Build history of the part. All positions in model axes, mm. Face numbers are marked on the shaded views. Round coordinates to 2 decimals unless told otherwise and drop trailing zeros. Write each loop counter-clockwise with the first axis right and the second up, starting at its lowest first coordinate (ties: lowest second). Pieces come first, ordered by that corner, then holes. Notation, with made-up numbers: M -3.75,60 L 33.25,60 A17 cw 33.25,79 Z; hole C 75.5,25.5 d4. An arc over 180 degrees is marked long. Use a Markdown table: item, result.
from build123d import *

# Parameters (mm, degrees)
SKETCH3_R          = 67.964535867
SKETCH3_R_2        = 37.5
CUT_EXTRUDE3_DEPTH = 10
SKETCH4_R          = 35.5
CUT_EXTRUDE4_DEPTH = 1
SKETCH6_R          = 2
CUT_EXTRUDE5_DEPTH = 10
SKETCH7_R          = 3.5
CUT_EXTRUDE6_DEPTH = 4
FILLET1_R          = 2


with BuildPart() as part:
    # Sketch1 → Revolve1 (revolve)
    with BuildSketch(Plane.XY):
        Polygon((-21, 11), (-60, 11), (-60, -8), (-21, -8), (-21, 0), (-16, 0), (-16, 4), (-21, 4), align=None)
    revolve(axis=Axis((0, 11, 0), (0, -1, 0)))

    # Sketch3 → Cut-Extrude3 (cut)
    with BuildSketch(Plane.XZ.offset(-11)):
        Circle(SKETCH3_R)
        with Locations(Location((0, 0, 0), (0, 0, 270))):
            Circle(SKETCH3_R_2, mode=Mode.SUBTRACT)
    extrude(amount=CUT_EXTRUDE3_DEPTH, mode=Mode.SUBTRACT)

    # Sketch4 → Cut-Extrude4 (cut)
    with BuildSketch(Plane.XZ.offset(8)):
        with Locations(Location((0, 0, 0), (0, 0, 270))):
            Circle(SKETCH4_R)
    extrude(amount=-CUT_EXTRUDE4_DEPTH, mode=Mode.SUBTRACT)

    # Sketch6 → Cut-Extrude5 (cut)
    with BuildSketch(Plane(origin=(0, 1, 0), x_dir=(1, 0, 0), z_dir=(0, 1, 0))):
        with Locations(Location((0, 54, 0), (0, 0, 270))):
            Circle(SKETCH6_R)
        with Locations(Location((38.183766184, 38.183766184, 0), (0, 0, 270))):
            Circle(SKETCH6_R)
        with Locations(Location((54, 0, 0), (0, 0, 270))):
            Circle(SKETCH6_R)
        with Locations(Location((38.183766184, -38.183766184, 0), (0, 0, 270))):
            Circle(SKETCH6_R)
        with Locations(Location((0, -54, 0), (0, 0, 270))):
            Circle(SKETCH6_R)
        with Locations(Location((-38.183766184, -38.183766184, 0), (0, 0, 270))):
            Circle(SKETCH6_R)
        with Locations(Location((-54, 0, 0), (0, 0, 270))):
            Circle(SKETCH6_R)
        with Locations(Location((-38.183766184, 38.183766184, 0), (0, 0, 270))):
            Circle(SKETCH6_R)
    extrude(amount=-CUT_EXTRUDE5_DEPTH, mode=Mode.SUBTRACT)

    # Sketch7 → Cut-Extrude6 (cut)
    with BuildSketch(Plane(origin=(0, 1, 0), x_dir=(1, 0, 0), z_dir=(0, 1, 0))):
        with Locations(Location((0, 54, 0), (0, 0, 270))):
            Circle(SKETCH7_R)
        with Locations(Location((38.183766184, 38.183766184, 0), (0, 0, 270))):
            Circle(SKETCH7_R)
        with Locations(Location((54, 0, 0), (0, 0, 270))):
            Circle(SKETCH7_R)
        with Locations(Location((38.183766184, -38.183766184, 0), (0, 0, 270))):
            Circle(SKETCH7_R)
        with Locations(Location((0, -54, 0), (0, 0, 270))):
            Circle(SKETCH7_R)
        with Locations(Location((-38.183766184, -38.183766184, 0), (0, 0, 270))):
            Circle(SKETCH7_R)
        with Locations(Location((-54, 0, 0), (0, 0, 270))):
            Circle(SKETCH7_R)
        with Locations(Location((-38.183766184, 38.183766184, 0), (0, 0, 270))):
            Circle(SKETCH7_R)
    extrude(amount=-CUT_EXTRUDE6_DEPTH, mode=Mode.SUBTRACT)

    # Fillet1
    fillet1_edges = [part.edges().sort_by_distance(p)[0] for p in [
        (0, 1, 37.5),
    ]]
    fillet(fillet1_edges, radius=FILLET1_R)


solid = part.part
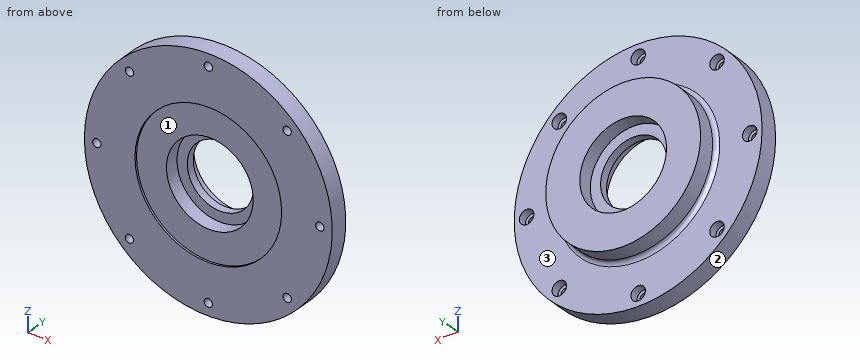
Q1. Cut at C-C on x = -54. Give the cut face in (y, z), and give its area (3 significant figures).
Response values:
| item | result |
|---|---|
| outline | M -8,-26.15 L 1,-26.15 L 1,-3.5 L -3,-3.5 L -3,-2 L -8,-2 Z; M -8,2 L -3,2 L -3,3.5 L 1,3.5 L 1,26.15 L -8,26.15 Z |
| area | 423 mm2 |
Q2. Cut at B-B on x = 0. Count the separate pieces of the cut face and the enclosed holes in it, and give its area (3 significant figures).
Response values:
| item | result |
|---|---|
| separate pieces | 4 |
| enclosed holes | 0 |
| area | 949 mm2 |
Q3. Cut at A-A on z = 54. Give the cut face in (x, y), and give its area (3 significant figures).
Response values:
| item | result |
|---|---|
| outline | M -26.15,-8 L -2,-8 L -2,-3 L -3.5,-3 L -3.5,1 L -26.15,1 Z; M 2,-8 L 26.15,-8 L 26.15,1 L 3.5,1 L 3.5,-3 L 2,-3 Z |
| area | 423 mm2 |
Q4. Drop flat-ended pins along their axis: P1, Ø2, axis at y = -3, z = -18, coming from the +X side; P2, Ø5, axis at y = 0.5, z = 37, coming from the +X side; P3, Ø2, axis at x = -13.5, z = 4, coming from the +Y side; P4, Ø3.5, axis at x = 38.5, z = 37.5, coming from the +Y side. Give the stop position or say it passes through.
Response values:
| item | result |
|---|---|
| P1 | stops at x = 57.54 |
| P2 | stops at x = 49.09 |
| P3 | passes through |
| P4 | stops at y = -3 |
Q5. Drill centre lines: L1, parallel to X at y = -4.1, z = 0; L2, parallel to Z at x = 3, y = 10; L3, parallel to Y at x = 37, z = 42. Where is each one in solid material? Low to high.
Response values:
| item | result |
|---|---|
| L1 | x = -60 to -56, -52 to -21, 21 to 52, 56 to 60 |
| L2 | z = -37.38 to -20.78, 20.78 to 37.38 |
| L3 | y = -8 to 1 |
Q6. Two-plate mould, pull along Z, no slides. Class the marked faces 1, 2 and 3: +Z half, -Z half, draft (parallel to the pull), parting line (faces both ways), or undercut.
Response values:
| item | result |
|---|---|
| face 1 | undercut |
| face 2 | parting line |
| face 3 | draft |
